Geometry: final body of the model. Coordinates: model frame, mm. A direction names the side the tool comes from. Give positions to 0.01 mm unless a question says otherwise; leave off trailing zeros. Loops run counter-clockwise (first coordinate to the right, second up) from the corner with the lowest first, then second, coordinate; pieces in that order, holes last. Notation, with made-up numbers: (-34, 19.25) -> (23, 19.25) arc R9 ccw to (23, 23.25) -> close; hole circle Ø5 at (36, -12.5). An arc over 180 degrees is marked (long way). Answer in a Markdown table with one row per item. Add a question column.
from build123d import *

# Parameters (mm, degrees)
SKETCH1_R           = 3.3782
SKETCH1_R_2         = 14.0335
SKETCH1_R_3         = 7.9375
SKETCH1_R_4         = 9.525
SKETCH1_R_5         = 4
BOSS_EXTRUDE2_DEPTH = 4.7625
CUT_EXTRUDE1_DEPTH  = 122.517222726
FILLET1_R           = 5.08


with BuildPart() as part:
    # Sketch1 → Boss-Extrude2 (new body)
    # profile 1 of 4: a face of its own
    with BuildSketch(Plane(origin=(0, 0, 0), x_dir=(1, 0, 0), z_dir=(0, 1, 0))):
        with BuildLine():
            ThreePointArc((-0.701449718, 27.635062977), (-8.547313483, 18.259236266), (-19.159429037, 24.329385209))
            Line((-19.159429037, 24.329385209), (-8.932978723, -3.305679376))
            ThreePointArc((-8.932978723, -3.305679376), (-1.67913708, 9.375826559), (9.525, 0))
            ThreePointArc((9.525, 0), (6.735192091, -6.735192091), (0, -9.525))
            Line((0, -9.525), (100.940182628, -14.019608589))
            ThreePointArc((100.940182628, -14.019608589), (87.638415083, 1.733479809), (104.396235267, 13.744819308))
            Line((104.396235267, 13.744819308), (-8.304416732, 36.964125856))
            ThreePointArc((-8.304416732, 36.964125856), (-2.842921118, 33.652465273), (-0.701449718, 27.635062977))
        make_face()
    # profile 2 of 4: a face of its own
    with BuildSketch(Plane(origin=(0, 0, 0), x_dir=(1, 0, 0), z_dir=(0, 1, 0))):
        with BuildLine():
            ThreePointArc((9.525, 0), (-1.67913708, 9.375826559), (-8.932978723, -3.305679376))
            ThreePointArc((-8.932978723, -3.305679376), (-5.442381324, -7.817039755), (0, -9.525))
            ThreePointArc((0, -9.525), (6.735192091, -6.735192091), (9.525, 0))
        make_face()
        with Locations(Location((0, 0, 0), (0, 0, 90))):
            Circle(SKETCH1_R, mode=Mode.SUBTRACT)
    # profile 3 of 4: a face of its own
    with BuildSketch(Plane(origin=(0, 0, 0), x_dir=(1, 0, 0), z_dir=(0, 1, 0))):
        with Locations((101.56444, 0)):
            Circle(SKETCH1_R_2)
        with Locations(Location((101.56444, 0, 0), (0, 0, 90))):
            Circle(SKETCH1_R_3, mode=Mode.SUBTRACT)
    # profile 4 of 4: a face of its own
    with BuildSketch(Plane(origin=(0, 0, 0), x_dir=(1, 0, 0), z_dir=(0, 1, 0))):
        with Locations((-10.226449718, 27.635062977)):
            Circle(SKETCH1_R_4)
        with Locations(Location((-10.226449718, 27.635062977, 0), (0, 0, 90))):
            Circle(SKETCH1_R_5, mode=Mode.SUBTRACT)
    extrude(amount=BOSS_EXTRUDE2_DEPTH)

    # Sketch2 → Cut-Extrude1 (cut, through all)
    with BuildSketch(Plane(origin=(0, 4.7625, 0), x_dir=(1, 0, 0), z_dir=(0, 1, 0))):
        with BuildLine():
            Line((92.787243401, 10.949883201), (-1.078567334, 30.28871572))
            ThreePointArc((-1.078567334, 30.28871572), (-2.569093415, 21.970213513), (-10.087484888, 18.111076743))
            Line((-10.087484888, 18.111076743), (-6.094283979, 7.320199983))
            ThreePointArc((-6.094283979, 7.320199983), (6.155929185, 7.26843593), (8.223542142, -4.806139786))
            Line((8.223542142, -4.806139786), (90.370654862, -8.463940958))
            ThreePointArc((90.370654862, -8.463940958), (87.638415083, 1.733479809), (92.787243401, 10.949883201))
        make_face()
    extrude(amount=-CUT_EXTRUDE1_DEPTH, mode=Mode.SUBTRACT)

    # Fillet1
    fillet1_edges = [part.edges().sort_by_distance(p)[0] for p in [
        (8.223542142, 2.38125, 4.806139786),
        (-6.094283979, 2.38125, -7.320199983),
        (-10.087484888, 2.38125, -18.111076743),
        (-1.078567334, 2.38125, -30.28871572),
        (92.787243401, 2.38125, -10.949883201),
        (90.370654862, 2.38125, 8.463940958),
    ]]
    fillet(fillet1_edges, radius=FILLET1_R)


solid = part.part
(1) Material intervals for line 1 along X through (y, z) = (2.75, 0) (3 decimals); line 2 along X through (y, z) = (0.8, -1); line 3 along X through (y, z) = (3.1, -11.5), sorted ascending. Write a range as from..to.
(2) Draft query along Z for faces 3 (the cylindrical face through (-2.7, 2.4, -21.8)), 4 (the cylindrical face through (115.45, 2.35, 2.02)), 5 (the cylindrical face through (86.444, 2.348, 6.464)), 6 (the flat face through (43, 0, 7)). Return one class per face: +Z half, -Z half, draft (parallel to the pull), parting line (faces both ways), or undercut.
(3) Cut plane A-A on x = 56. Return the cut outline in (y, z).
(4) Pin query (flat end, axial travel): pin 1 Ø7 at (x, z) = (-10.23, -27.64) entering from -Y; pin 2 Ø1.5 at (y, z) = (1.5, -4.5) entering from +X; pin 3 Ø1.5 at (x, y) = (69.5, 0.5) entering from -Z; pin 4 Ø1.5 at (y, z) = (2.5, -1) entering from -X. Return the tip coordinate at first contact, or that it passes through.
(5) Reachability of faces 1 (the flat face through (48.8, 2.3, -25.2)), 2 (the cylindrical face through (10.9, 2.35, 3.48)) from +Z, -Z, +X, -X, +Y, -Y: full face, straight path, thin tool, end or side. Return the list, or none.
(6) Cut plane B-B on y = 1.3. State how many separate pieces and enclosed holes the cut face has, then the cut area to 3 significant figures.
Answer list:
| question | item | result |
|---|---|---|
| 1 | line 1 | x = -10.156..-3.378, 3.378..9.525, 87.531..93.627, 109.502..115.598 |
| 1 | line 2 | x = -10.53..-3.23, 3.23..9.47, 87.57..93.69, 109.44..115.56 |
| 1 | line 3 | x = -14.41..-7.52, 87.23..109.61 |
| 2 | face 3 | undercut |
| 2 | face 4 | parting line |
| 2 | face 5 | undercut |
| 2 | face 6 | draft |
| 3 | outline | (0, -23.72) -> (4.76, -23.72) -> (4.76, -18.53) -> (0, -18.53) -> close; (0, 6.93) -> (4.76, 6.93) -> (4.76, 12.02) -> (0, 12.02) -> close |
| 4 | pin 1 | passes through |
| 4 | pin 2 | stops at x = 115.09 |
| 4 | pin 3 | stops at z = -21.09 |
| 4 | pin 4 | stops at x = -10.8 |
| 5 | face 1 | -Z, +X, +Y, -Y |
| 5 | face 2 | +Y, -Y |
| 6 | separate pieces | 1 |
| 6 | enclosed holes | 4 |
| 6 | area | 2,020 mm² |
